Answer from the drawing. Dimensions are ordinates in mm from the lowest x, y and z of the part. A direction names the side the tool comes from. Coordinates: 2 decimals unless noted, no trailing zeros. Write each loop counter-clockwise with the first axis right and the second up, starting at its lowest first coordinate (ties: lowest second). Pieces come first, ordered by that corner, then holes. Notation, with made-up numbers: (-34.5, 12) -> (10.5, 12) arc R4 cw to (10.5, 16) -> close; hole circle Ø3 at (47.5, 5.5). An arc over 180 degrees is marked (long way). One line per item, written item: value. Start each with the question number.
1. Find section C-C, the plane y = 3.5. Write down the section's boundary in (x, z), and give its area (3 significant figures).
2. Find section D-D, the plane x = 42.5. Write down the section's boundary in (y, z), and give its area (3 significant figures).
3. For the marked faces 1, 2 and 3, determine the directions among +Z, -Z, +X, -X, +Y, -Y from which every point of the face is accessible in a straight line to the end or side of a thin tool.
4. Find section B-B, the plane x = 35. Write down the section's boundary in (y, z), and give its area (3 significant figures).
5. Given P1, Ø1.6, axis at y = 1, z = 2.5, coming from the +X side; P2, Ø1.5, axis at x = 3.5, z = 1.5, coming from the +Y side; P3, Ø2, axis at y = 7.5, z = 2.5, coming from the -X side, each flat-ended and moving along its own axis, determine where each tip first touches the part or whether it passes through.
6. Find section A-A, the plane z = 3.45. Write down the section's boundary in (x, y).
7. Consider line 1 along X through (y, z) = (5.25, 1.15); line 2 along Y through (x, z) = (32, 4.55); line 3 along X through (y, z) = (6.5, 0.4). Determine where each line is inside the solid, lowest interval first.
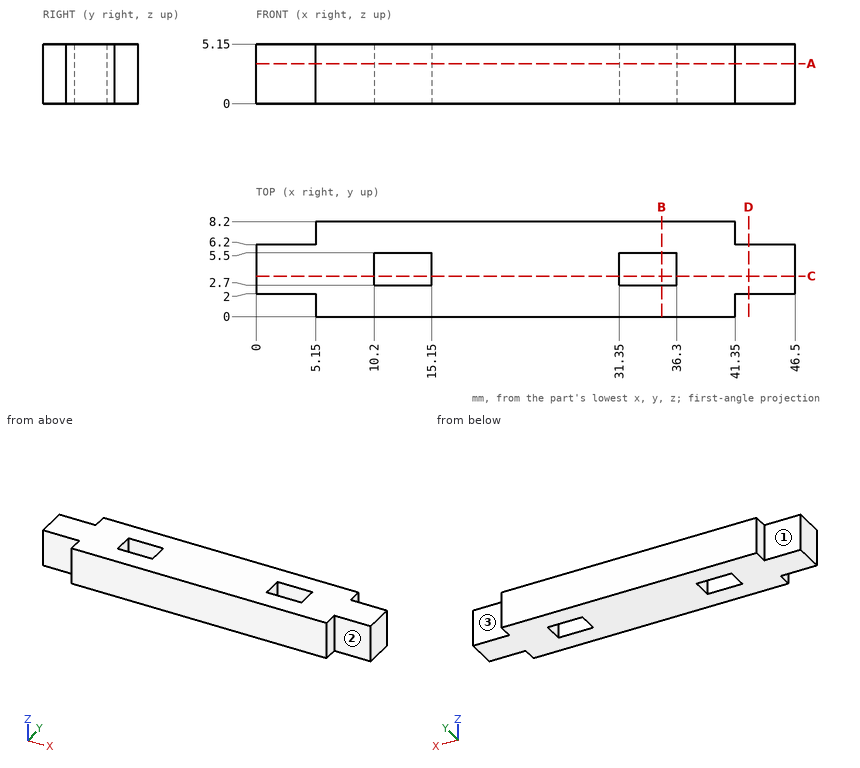
Answer block:
1. outline: (0, 0) -> (10.2, 0) -> (10.2, 5.15) -> (0, 5.15) -> close; (15.15, 0) -> (31.35, 0) -> (31.35, 5.15) -> (15.15, 5.15) -> close; (36.3, 0) -> (46.5, 0) -> (46.5, 5.15) -> (36.3, 5.15) -> close
1. area: 188 mm2
2. outline: (2, 0) -> (6.2, 0) -> (6.2, 5.15) -> (2, 5.15) -> close
2. area: 21.6 mm2
3. face 1: +Z, -Z, -X, +Y
3. face 2: +Z, -Z, +X, -Y
3. face 3: +Z, -Z, +X, +Y
4. outline: (0, 0) -> (2.7, 0) -> (2.7, 5.15) -> (0, 5.15) -> close; (5.5, 0) -> (8.2, 0) -> (8.2, 5.15) -> (5.5, 5.15) -> close
4. area: 27.8 mm2
5. P1: stops at x = 41.35
5. P2: stops at y = 6.2
5. P3: stops at x = 5.15
6. outline: (0, 2) -> (5.15, 2) -> (5.15, 0) -> (41.35, 0) -> (41.35, 2) -> (46.5, 2) -> (46.5, 6.2) -> (41.35, 6.2) -> (41.35, 8.2) -> (5.15, 8.2) -> (5.15, 6.2) -> (0, 6.2) -> close; hole (10.2, 2.7) -> (15.15, 2.7) -> (15.15, 5.5) -> (10.2, 5.5) -> close; hole (31.35, 2.7) -> (36.3, 2.7) -> (36.3, 5.5) -> (31.35, 5.5) -> close
7. line 1: x = 0 to 10.2, 15.15 to 31.35, 36.3 to 46.5
7. line 2: y = 0 to 2.7, 5.5 to 8.2
7. line 3: x = 5.15 to 41.35
